Autodesk Inventor part; units mm, degrees
ref_plane "YZ Plane" through (0, 0, 0) normal (1, 0, 0) x (0, 1, 0)
ref_plane "XZ Plane" through (0, 0, 0) normal (0, 1, 0) x (-1, 0, 0)
ref_plane "XY Plane" through (0, 0, 0) normal (0, 0, 1) x (1, 0, 0)
sketch "Sketch1" plane through (0, 0, 0) normal (0, 0, 1) x (1, 0, 0)
  line L0 (0, 0) -> (83, 0)
  line L1 (83, 0) -> (83, 139.7)
  line L2 (83, 139.7) -> (0, 139.7)
  line L3 (0, 139.7) -> (0, 0)
  dimension "d0" = 83
  dimension "d1" = 139.7
extrude "Extrusion1" add sketch "Sketch1" along normal blind 59.1
sketch "Sketch2" plane through (0, 139.7, 0) normal (0, 1, 0) x (1, 0, 0)
  line L0 (0, -9) -> (47.7, -9)
  line L1 (47.7, -9) -> (47.7, -12)
  line L2 (47.7, -12) -> (0, -12)
  line L3 (0, -12) -> (0, -9)
  line L4 (83, 0) -> (0, 0)
  line L5 (13, -12) -> (16, -12)
  line L6 (16, -12) -> (16, -21.7)
  line L7 (16, -21.7) -> (13, -21.7)
  line L8 (13, -21.7) -> (13, -12)
  line L9 (0, 0) -> (0, -59.1)
  line L10 (29, -12) -> (32, -12)
  line L11 (32, -12) -> (32, -21.7)
  line L12 (32, -21.7) -> (29, -21.7)
  line L13 (29, -21.7) -> (29, -12)
  dimension "d4" = 3
  dimension "d5" = 47.7
  dimension "d6" = 9
  dimension "d7" = 9.7
  dimension "d8" = 3
  dimension "d9" = 13
  dimension "d10" = 3
  dimension "d11" = 9.7
  dimension "d12" = 29
extrude "Extrusion2" add sketch "Sketch2" along normal blind 11.37
sketch "Sketch3" plane through (0, 0, 0) normal (0, -1, 0) x (1, 0, 0)
  line L0 (83, 0) -> (0, 0)
  line L1 (0, 9) -> (47.7, 9)
  line L2 (47.7, 9) -> (47.7, 12)
  line L3 (47.7, 12) -> (0, 12)
  line L4 (0, 12) -> (0, 9)
  line L5 (13, 12) -> (16, 12)
  line L6 (16, 12) -> (16, 21.7)
  line L7 (16, 21.7) -> (13, 21.7)
  line L8 (13, 21.7) -> (13, 12)
  line L9 (0, 0) -> (0, 59.1)
  line L10 (29, 12) -> (32, 12)
  line L11 (32, 12) -> (32, 21.7)
  line L12 (32, 21.7) -> (29, 21.7)
  line L13 (29, 21.7) -> (29, 12)
extrude "Extrusion3" add sketch "Sketch3" along normal blind 11.37
fillet "Fillet1" radius 5 4 edges at (0, 151.07, 10.5) (47.7, 151.07, 10.5) (0, -11.37, 10.5) (47.7, -11.37, 10.5)
chamfer "Chamfer1" distance 5 angle 45 4 edges at (30.5, -11.37, 21.7) (14.5, -11.37, 21.7) (30.5, 151.07, 21.7) (14.5, 151.07, 21.7)
sketch "Sketch5" plane through (47.7, 0, 9) normal (0, 0, -1) x (-1, 0, 0)
  circle A0 centre (6, 146.47) radius 2.5
  circle A1 centre (41.7, 146.47) radius 2.5
  circle A2 centre (6, -6.77) radius 2.5
  circle A3 centre (41.7, -6.77) radius 2.5
  line L0 (47.7, 0) -> (47.7, -6.37)
  line L1 (0, 0) -> (0, -6.37)
  line L2 (0, 139.7) -> (0, 146.07)
  line L3 (47.7, 139.7) -> (47.7, 146.07)
  line L4 (5, 151.07) -> (42.7, 151.07)
  line L5 (42.7, -11.37) -> (5, -11.37)
  dimension "d30" = 5
  dimension "d31" = 5
  dimension "d32" = 5
  dimension "d33" = 5
  dimension "d34" = 6
  dimension "d35" = 6
  dimension "d36" = 6
  dimension "d37" = 6
  dimension "d38" = 4.6
  dimension "d39" = 4.6
  dimension "d40" = 4.6
  dimension "d41" = 4.6
extrude "Extrusion4" cut sketch "Sketch5" against normal up to next
properties part number "Battery" material "Aluminum 6061-AHC"
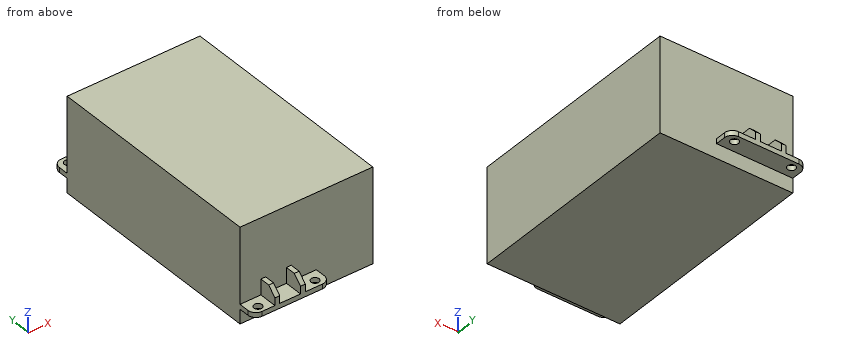
Work out the finished part from the listing and answer in its coordinate system (mm). Round coordinates to 2 decimals unless told otherwise and drop trailing zeros. Loops run counter-clockwise (first coordinate to the right, second up) from the corner with the lowest first, then second, coordinate; pieces in that order, holes last.
(1) The part is cut by section C-C, the plane z = 29. Give the vertices of the cut face in (x, y).
Computed values:
outline: (0, 0) - (83, 0) - (83, 139.7) - (0, 139.7) - close
(2) Each of these flat-tipped pins is pushed along its axis until it touches: P1, Ø5, axis at x = 60.5, z = 51.5, coming from the -Y side; P2, Ø9, axis at x = 18.5, y = 148, coming from the -Z side; P3, Ø3.5, axis at x = 43.5, y = 146, coming from the +Z side; P4, Ø4, axis at x = 6, y = 146.47, coming from the -Z side. Where does it stop, or does it pass through?
Computed values:
P1: stops at y = 0
P2: stops at z = 9
P3: stops at z = 12
P4: passes through
(3) Find the intervals of material crossed by L1, parallel to Y at x = 6, z = 10.75; L2, parallel to X at y = 146.47, z = 11.4; L3, parallel to Y at x = 79, z = 44, in increasing order.
Computed values:
L1: y = -11.37 to -9.27, -4.27 to 143.97, 148.97 to 151.07
L2: x = 0.02 to 3.5, 8.5 to 39.2, 44.2 to 47.68
L3: y = 0 to 139.7
(4) The part is cut by section A-A, the plane z = 14.5. Give the vertices of the cut face in (x, y).
Computed values:
outline: (0, 0) - (13, 0) - (13, -11.37) - (16, -11.37) - (16, 0) - (29, 0) - (29, -11.37) - (32, -11.37) - (32, 0) - (83, 0) - (83, 139.7) - (32, 139.7) - (32, 151.07) - (29, 151.07) - (29, 139.7) - (16, 139.7) - (16, 151.07) - (13, 151.07) - (13, 139.7) - (0, 139.7) - close
(5) The part is cut by section B-B, the plane x = 51.5. Give the vertices of the cut face in (y, z).
Computed values:
outline: (0, 0) - (139.7, 0) - (139.7, 59.1) - (0, 59.1) - close
